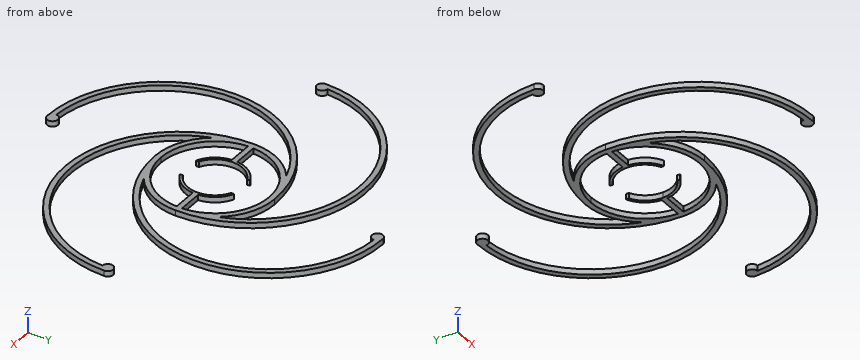
from build123d import *

# Parameters (mm, degrees)
F1_DEPTH   = 1
F1_FACE_W  = 1
F1_FACE_H  = 1
F1_FACE1_W = 1
F1_FACE1_H = 1
F1_FACE2_W = 1
F1_FACE2_H = 1
F1_FACE3_W = 1
F1_FACE3_H = 1


# Not quite as in the source:
# - a feature names something its author has since deleted; it is built from what else it names


with BuildPart() as f1:
    # F0 (on Top) → F1 (new body)
    with BuildSketch(Plane.XY):
        with BuildLine():
            ThreePointArc((8.95, 6.3951153234), (9.735754356, 3.2403703492), (10, 0))
            ThreePointArc((10, 0), (9.9968982101, -0.2490505519), (9.9875947645, -0.4979466032))
            ThreePointArc((9.9875947645, -0.4979466032), (6.8927691811, -7.2449798493), (0, -10))
            ThreePointArc((0, -10), (3.2403703492, -9.735754356), (6.3951153234, -8.95))
            ThreePointArc((6.3951153234, -8.95), (9.7812644519, -5.0325804237), (11, 0))
            ThreePointArc((11, 0), (10.474970167, 3.3578266781), (8.95, 6.3951153234))
        make_face()
        with BuildLine():
            ThreePointArc((9.9875947645, 0.4979466032), (9.9968982101, 0.2490505519), (10, 0))
            ThreePointArc((10, 0), (9.735754356, 3.2403703492), (8.95, 6.3951153234))
            ThreePointArc((8.95, 6.3951153234), (5.0325804237, 9.7812644519), (0, 11))
            ThreePointArc((0, 11), (-3.3578266781, 10.474970167), (-6.3951153234, 8.95))
            ThreePointArc((-6.3951153234, 8.95), (-3.2403703492, 9.735754356), (0, 10))
            ThreePointArc((0, 10), (6.8927691811, 7.2449798493), (9.9875947645, 0.4979466032))
        make_face()
        with BuildLine():
            ThreePointArc((-30, 0), (-13.2403703492, 19.735754356), (8.95, 6.3951153234))
            ThreePointArc((8.95, 6.3951153234), (10.474970167, 3.3578266781), (11, 0))
            ThreePointArc((11, 0), (-10, 21), (-31, 0))
            Line((-31, 0), (-30, 0))
        make_face()
        with BuildLine():
            ThreePointArc((-9.9875233888, 0.4993761694), (-6.8922506595, 7.2454731279), (0, 10))
            ThreePointArc((0, 10), (-3.2403703492, 9.735754356), (-6.3951153234, 8.95))
            ThreePointArc((-6.3951153234, 8.95), (-9.7812644519, 5.0325804237), (-11, 0))
            ThreePointArc((-11, 0), (-10.474970167, -3.3578266781), (-8.95, -6.3951153234))
            ThreePointArc((-8.95, -6.3951153234), (-9.735754356, -3.2403703492), (-10, 0))
            ThreePointArc((-10, 0), (-9.9968803606, 0.2497660027), (-9.9875233888, 0.4993761694))
        make_face()
        with BuildLine():
            ThreePointArc((6.3951153234, -8.95), (3.2403703492, -9.735754356), (0, -10))
            ThreePointArc((0, -10), (-6.8922506595, -7.2454731279), (-9.9875233888, -0.4993761694))
            ThreePointArc((-9.9875233888, -0.4993761694), (-9.9968803606, -0.2497660027), (-10, 0))
            ThreePointArc((-10, 0), (-9.735754356, -3.2403703492), (-8.95, -6.3951153234))
            ThreePointArc((-8.95, -6.3951153234), (-5.0325804237, -9.7812644519), (0, -11))
            ThreePointArc((0, -11), (3.3578266781, -10.474970167), (6.3951153234, -8.95))
        make_face()
        with BuildLine():
            ThreePointArc((-6.3951153234, 8.95), (-3.3578266781, 10.474970167), (0, 11))
            ThreePointArc((0, 11), (-21, -10), (0, -31))
            Line((0, -31), (0, -30))
            ThreePointArc((0, -30), (-19.735754356, -13.2403703492), (-6.3951153234, 8.95))
        make_face()
        with BuildLine():
            ThreePointArc((0, 30), (19.735754356, 13.2403703492), (6.3951153234, -8.95))
            ThreePointArc((6.3951153234, -8.95), (3.3578266781, -10.474970167), (0, -11))
            ThreePointArc((0, -11), (21, 10), (0, 31))
            Line((0, 31), (0, 30))
        make_face()
        with BuildLine():
            ThreePointArc((-8.95, -6.3951153234), (-10.474970167, -3.3578266781), (-11, 0))
            ThreePointArc((-11, 0), (10, -21), (31, 0))
            Line((31, 0), (30, 0))
            ThreePointArc((30, 0), (13.2403703492, -19.735754356), (-8.95, -6.3951153234))
        make_face()
        with BuildLine():
            ThreePointArc((5.5, 0), (5.4943502571, 0.2492293164), (5.4774126356, 0.4979466032))
            ThreePointArc((5.4774126356, 0.4979466032), (4.4763336759, 3.1956903514), (2.25, 5.018714975))
            Line((2.25, 5.018714975), (2.25, 4.4651427749))
            ThreePointArc((2.25, 4.4651427749), (4.2573465915, 2.6220221204), (5, 0))
            ThreePointArc((5, 0), (4.2573465915, -2.6220221204), (2.25, -4.4651427749))
            Line((2.25, -4.4651427749), (2.25, -5.018714975))
            ThreePointArc((2.25, -5.018714975), (4.4763336759, -3.1956903514), (5.4774126356, -0.4979466032))
            ThreePointArc((5.4774126356, -0.4979466032), (5.4943502571, -0.2492293164), (5.5, 0))
        make_face()
        with BuildLine():
            ThreePointArc((9.9875947645, -0.4979466032), (9.9968982101, -0.2490505519), (10, 0))
            ThreePointArc((10, 0), (9.9968982101, 0.2490505519), (9.9875947645, 0.4979466032))
            Line((9.9875947645, 0.4979466032), (5.4774126356, 0.4979466032))
            ThreePointArc((5.4774126356, 0.4979466032), (5.4943502571, 0.2492293164), (5.5, 0))
            ThreePointArc((5.5, 0), (5.4943502571, -0.2492293164), (5.4774126356, -0.4979466032))
            Line((5.4774126356, -0.4979466032), (9.9875947645, -0.4979466032))
        make_face()
        with BuildLine():
            ThreePointArc((-2.25, 5.018714975), (-4.4761862714, 3.1958968168), (-5.4773666772, 0.4984518873))
            ThreePointArc((-5.4773666772, 0.4984518873), (-5.5, 0), (-5.4773666772, -0.4984518873))
            ThreePointArc((-5.4773666772, -0.4984518873), (-4.4761862714, -3.1958968168), (-2.25, -5.018714975))
            Line((-2.25, -5.018714975), (-2.25, -4.4651427749))
            ThreePointArc((-2.25, -4.4651427749), (-5, 0), (-2.25, 4.4651427749))
            Line((-2.25, 4.4651427749), (-2.25, 5.018714975))
        make_face()
        with BuildLine():
            Line((-5.4773666772, 0.4984518873), (-9.9875233888, 0.4993761694))
            ThreePointArc((-9.9875233888, 0.4993761694), (-9.9968803606, 0.2497660027), (-10, 0))
            ThreePointArc((-10, 0), (-9.9968803606, -0.2497660027), (-9.9875233888, -0.4993761694))
            Line((-9.9875233888, -0.4993761694), (-5.4773666772, -0.4984518873))
            ThreePointArc((-5.4773666772, -0.4984518873), (-5.5, 0), (-5.4773666772, 0.4984518873))
        make_face()
    extrude(amount=F1_DEPTH)

    # F1_face (on face) → F2 (revolve)
    with BuildSketch(Plane(origin=(-30.5, 0, 0.5), x_dir=(1, 0, 0), z_dir=(0, -1, 0))):
        Rectangle(F1_FACE_W, F1_FACE_H)
    revolve(axis=Axis((-30, 0, 0.5), (0, 0, -1)))

    # F1_face1 (on face) → F3 (revolve)
    with BuildSketch(Plane(origin=(0, -30.5, 0.5), x_dir=(0, 1, 0), z_dir=(1, 0, 0))):
        Rectangle(F1_FACE1_W, F1_FACE1_H)
    revolve(axis=Axis((0, -30, 0.5), (0, 0, -1)))

    # F1_face2 (on face) → F4 (revolve)
    with BuildSketch(Plane(origin=(30.5, 0, 0.5), x_dir=(-1, 0, 0), z_dir=(0, 1, 0))):
        Rectangle(F1_FACE2_W, F1_FACE2_H)
    revolve(axis=Axis((30, 0, 0.5), (0, 0, -1)))

    # F1_face3 (on face) → F5 (revolve)
    with BuildSketch(Plane(origin=(0, 30.5, 0.5), x_dir=(0, -1, 0), z_dir=(-1, 0, 0))):
        Rectangle(F1_FACE3_W, F1_FACE3_H)
    revolve(axis=Axis((0, 30, 0.5), (0, 0, -1)))


solid = f1.part
For this review, take the finished solid that the model builds, in its own axes (mm). Round coordinates to 2 decimals unless told otherwise and drop trailing zeros. Order: outer loops, then holes, each group sorted by start corner. A loop starts at its lowest first (then second) coordinate and runs counter-clockwise, first axis right, second up. Notation, with made-up numbers: (-32.5, 30) -> (3.5, 30) arc R20 cw to (3.5, 59) -> close; hole circle Ø2 at (33, -15.5). An arc over 180 degrees is marked (long way). Write item = value, one per line. Start each with the question number.
1) Insertion check: pin 1 (3 mm diameter, centred on x = 11, y = -1.5, fed in from +Z); pin 2 (0.6 mm diameter, centred on y = -4.5, z = 0.5, fed in from -X). Each pin has a flat end and moves straight along its axis. Give the tip position at first contact, or say it passes through.
2) Take a section at A-A on y = -8. State the section outline as (x, z) points, plus the area to 3 significant figures.
3) To check wall thickness, follow line 1 (Y direction, x = 6, z = 0.05); line 2 (Y direction, x = -17, z = 0.15) (3 decimals); line 3 (X direction, y = 15.5, z = 0.1). State the ranges of each line that lie inside material, in increasing order. Write a range as from..to.
4) Take a section at B-B on x = -26. State the section outline as (y, z) points, plus the area to 3 significant figures.
Verdict:
q1.pin_1 = 1
q1.pin_2 = -20.35
q2.outline = (-20.9, 0) -> (-19.9, 0) -> (-19.9, 1) -> (-20.9, 1) -> close; (-9.42, 0) -> (-8.33, 0) -> (-8.33, 1) -> (-9.42, 1) -> close; (-7.55, 0) -> (-6, 0) -> (-6, 1) -> (-7.55, 1) -> close; (6, 0) -> (7.55, 0) -> (7.55, 1) -> (6, 1) -> close; (8.72, 0) -> (10.82, 0) -> (10.82, 1) -> (8.72, 1) -> close; (28.33, 0) -> (29.42, 0) -> (29.42, 1) -> (28.33, 1) -> close
q2.area = 8.38 mm2
q3.line_1 = -20.62..-19.6, -10.12..-8, -0.5..0.5, 8..9.22, 12..13.6, 29.08..30.12
q3.line_2 = -22.329..-20.536, 0.536..2.329, 18.735..19.799
q3.line_3 = -24.17..-22.64, 2.64..4.17, 19.23..20.27
q4.outline = (12, 0) -> (13.6, 0) -> (13.6, 1) -> (12, 1) -> close
q4.area = 1.60 mm2
